For this review, take the finished solid that the model builds, in its own axes (mm). Face numbers are marked on the shaded views. A direction names the side the tool comes from. Round coordinates to 2 decimals unless told otherwise and drop trailing zeros. Write each loop counter-clockwise with the first axis right and the second up, starting at its lowest first coordinate (ties: lowest second). Pieces come first, ordered by that corner, then holes. Notation, with made-up numbers: (-23, -14) -> (-8, -14) arc R16 ccw to (-8, 3) -> close; hole circle Ø8 at (-24.75, -1). An arc over 180 degrees is marked (long way). Write item = value, one per line. Start each with the question number.
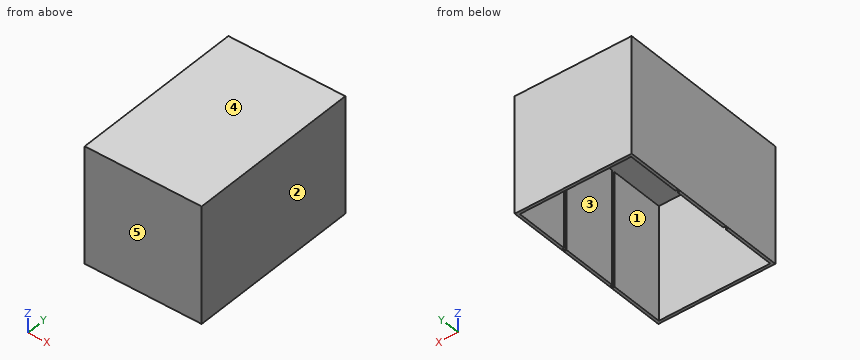
```python
from build123d import *

# Parameters (mm, degrees)
SKETCH1_W           = 500
SKETCH1_H           = 750
BOSS_EXTRUDE1_DEPTH = 500
SKETCH2_W           = 476
SKETCH2_H           = 726
CUT_EXTRUDE1_DEPTH  = 488
SKETCH3_W           = 6
SKETCH3_H           = 14
CUT_EXTRUDE2_DEPTH  = 488


with BuildPart() as part:
    # Sketch1 → Boss-Extrude1 (new body)
    with BuildSketch(Plane.XY):
        with Locations((250, 375)):
            Rectangle(SKETCH1_W, SKETCH1_H)
    extrude(amount=BOSS_EXTRUDE1_DEPTH)

    # Sketch2 → Cut-Extrude1 (cut)
    with BuildSketch(Plane(origin=(0, 0, 0), x_dir=(-1, 0, 0), z_dir=(0, 0, -1))):
        with Locations((-250, 375)):
            Rectangle(SKETCH2_W, SKETCH2_H)
    extrude(amount=-CUT_EXTRUDE1_DEPTH, mode=Mode.SUBTRACT)

    # Sketch3 → Cut-Extrude2 (cut)
    with BuildSketch(Plane(origin=(0, 0, 0), x_dir=(-1, 0, 0), z_dir=(0, 0, -1))):
        with Locations((-491, 250)):
            Rectangle(SKETCH3_W, SKETCH3_H)
        with Locations((-491, 500)):
            Rectangle(SKETCH3_W, SKETCH3_H)
        with Locations((-9, 500)):
            Rectangle(SKETCH3_W, SKETCH3_H)
        with Locations((-9, 250)):
            Rectangle(SKETCH3_W, SKETCH3_H)
    extrude(amount=-CUT_EXTRUDE2_DEPTH, mode=Mode.SUBTRACT)


solid = part.part
```
1. Clearance check with a flat-ended pin moving along its axis: pin 1 Ø1 at (x, y) = (100, 391) entering from -Z. State where the tip first meets the part, or that it passes through.
2. Draft analysis for pull direction Y (two halves, no side actions). For the marked faces 3, 4 and 5, state which applies: +Y half, -Y half, draft (parallel to the pull), parting line (faces both ways), or undercut.
3. Machinability: for the marked faces 1 and 2, which of the approach directions +Z, -Z, +X, -X, +Y, -Y give a long, thin tool a straight path to every point of the face, cutting with its end or side? Answer none if there is none.
4. Consider section C-C, the plane x = 152. Give the boundary of the cut face in (y, z).
5. Consider section B-B, the plane z = 124. Give the boundary of the cut face in (x, y).
6. Wall thickness on L1, parallel to X at y = 505, z = 391.5; L2, parallel to Y at x = 367, z = 422.5; L3, parallel to X at y = 162.5, z = 228.5: over which ranges is each line inside the solid? List them lowest first. Write a range as from..to.
7. Consider section A-A, the plane y = 449.5. Give the boundary of the cut face in (x, z), then the cut area to 3 significant figures.
Outcome:
q1.pin_1 = 488
q2.face_3 = undercut
q2.face_4 = draft
q2.face_5 = -Y half
q3.face_1 = -Z
q3.face_2 = +Z, -Z, +X, +Y, -Y
q4.outline = (0, 0) -> (12, 0) -> (12, 488) -> (738, 488) -> (738, 0) -> (750, 0) -> (750, 500) -> (0, 500) -> close
q5.outline = (0, 0) -> (500, 0) -> (500, 750) -> (0, 750) -> close; hole (6, 243) -> (12, 243) -> (12, 12) -> (488, 12) -> (488, 243) -> (494, 243) -> (494, 257) -> (488, 257) -> (488, 493) -> (494, 493) -> (494, 507) -> (488, 507) -> (488, 738) -> (12, 738) -> (12, 507) -> (6, 507) -> (6, 493) -> (12, 493) -> (12, 257) -> (6, 257) -> close
q6.L1 = 0..6, 494..500
q6.L2 = 0..12, 738..750
q6.L3 = 0..12, 488..500
q7.outline = (0, 0) -> (12, 0) -> (12, 488) -> (488, 488) -> (488, 0) -> (500, 0) -> (500, 500) -> (0, 500) -> close
q7.area = 17,700 mm2
